Part print with two shaded views. Sizes in mm from the minimum x, y, z corner. A direction names the side the tool comes from. Coordinates: 2 decimals unless noted, no trailing zeros. Order: outer loops, then holes, each group sorted by start corner. A loop starts at its lowest first (then second) coordinate and runs counter-clockwise, first axis right, second up. Notation, with made-up numbers: M 88,39 L 140,39 A13 ccw 140,63 Z; hole C 87.5,-20.5 d2. An arc over 180 degrees is marked long. Answer in a Markdown table with one row per item. Add a question column.
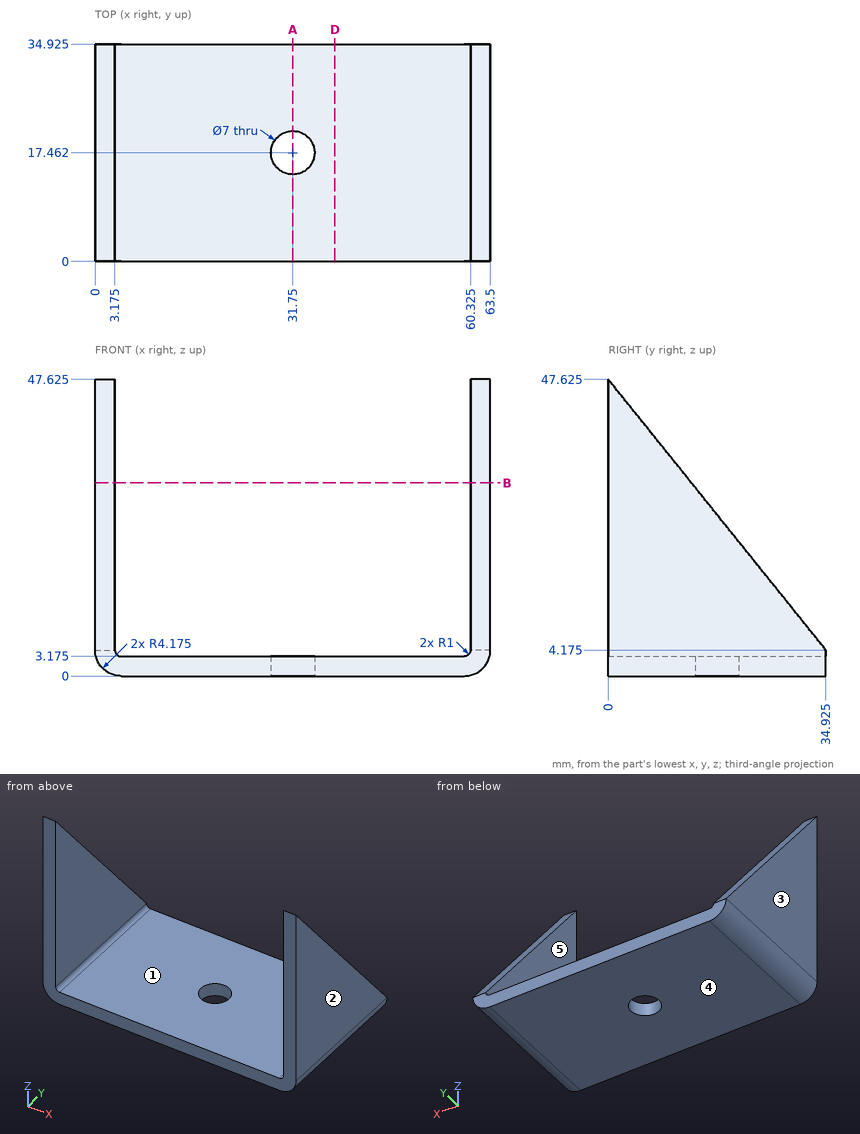
(1) Slice it at A-A (x = 31.75). List the corners of the cut face in (y, z) (1 decimal).
(2) Pull direction X, two halves, no side cores. Call the marked faces 3, 4 and 5: pulls with the +X half, pulls with the -X half, needs draft (parallel to the pull), parting line crosses it, or undercut.
(3) 3-axis set-ups, long thin cutter, end or side, ignore diameter. For the marked faces 1 and 2: which of +Z, -Z, +X, -X, +Y, -Y reach the whole face in a straight line?
(4) Drop a flat-ended pin along its axis: P1, Ø1, axis at x = 55, y = 16.5, coming from the +Z side (1 decimal). Give the stop position or say it passes through.
(5) Slice it at D-D (x = 38.5). List the corners of the cut face in (y, z) (1 decimal).
(6) Wall check: line 1 (X direction, y = 7, z = 24.5) (1 decimal); line 2 (Y direction, x = 31.75, z = 1.1) (1 decimal); line 3 (Z direction, x = 17, y = 16.5) (1 decimal). Give the ranges that are in metal, low to high.
(7) Slice it at B-B (z = 31). List the corners of the cut face in (x, y) (1 decimal).
Computed:
| question | item | result |
|---|---|---|
| 1 | outline | M 0,0 L 14,0 L 14,3.2 L 0,3.2 Z; M 21,0 L 34.9,0 L 34.9,3.2 L 21,3.2 Z |
| 2 | face 3 | pulls with the -X half |
| 2 | face 4 | needs draft |
| 2 | face 5 | undercut |
| 3 | face 1 | +Z, +Y, -Y |
| 3 | face 2 | +Z, -Z, +X, +Y, -Y |
| 4 | P1 | stops at z = 3.2 |
| 5 | outline | M 0,0 L 34.9,0 L 34.9,3.2 L 0,3.2 Z |
| 6 | line 1 | x = 0 to 3.2, 60.3 to 63.5 |
| 6 | line 2 | y = 0 to 14, 21 to 34.9 |
| 6 | line 3 | z = 0 to 3.2 |
| 7 | outline | M 0,0 L 3.2,0 L 3.2,13.4 L 0,13.4 Z; M 60.3,0 L 63.5,0 L 63.5,13.4 L 60.3,13.4 Z |
